Model file for the job. Use its own axes, mm. Give positions to 0.01 mm unless a question says otherwise; leave off trailing zeros. Loops run counter-clockwise (first coordinate to the right, second up) from the corner with the lowest first, then second, coordinate; pieces in that order, holes last. Notation, with made-up numbers: M 69,2.5 L 112,2.5 A28 ccw 112,33.5 Z; hole C 79,50 d2. An arc over 180 degrees is marked long. Use CSV: the item, a comma, the result in double quotes. Start each with the question number.
(1) Flat gauge pins, fed straight in: P1, Ø3, axis at x = 3, y = 407, coming from the -Z side; P2, Ø1.5, axis at x = 4.5, y = 323, coming from the -Z side; P3, Ø2, axis at x = 1, y = 427, coming from the -Z side. Where does each tip first touch, or does it go through?
(2) Slice it at D-D on z = 72.5. List the corners of the cut face in (x, y).
(3) Wall check: line 1 along Y through (x, z) = (2, 64); line 2 along Y through (x, z) = (0.5, 52); line 3 along Z through (x, y) = (1, 267.5). Give the ranges that are in metal, low to high. Write a range as from..to.
(4) Slice it at A-A on x = 5. List the corners of the cut face in (y, z).
(5) Slice it at B-B on z = 31.5. List the corners of the cut face in (x, y), and give its area (3 significant figures).
(6) Slice it at C-C on y = 269. List the corners of the cut face in (x, z).
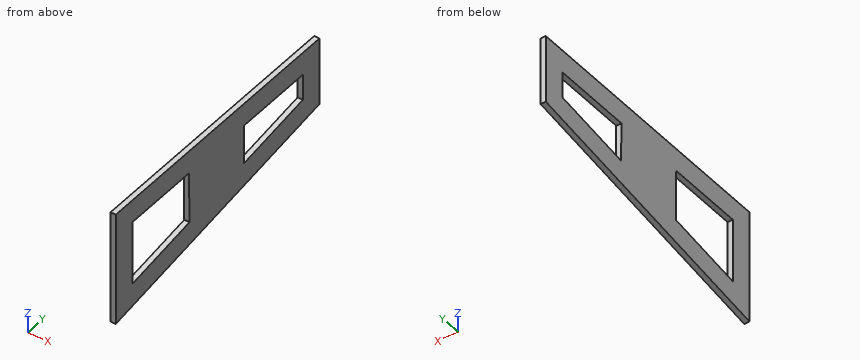
```python
from build123d import *

# Parameters (mm, degrees)
F1_DEPTH = 7


with BuildPart() as f1:
    # F0 (on Right) → F1 (new body)
    with BuildSketch(Plane.YZ):
        Polygon((599.109616, 110.551124), (232.423452, 105.89446), (232.423452, -44.10554), (599.109616, 20.551124), align=None)
        Polygon((262.423452, -8.352933), (262.423452, 76.27302), (364.232124, 77.565921), (365.093333, 9.750538), align=None, mode=Mode.SUBTRACT)
        Polygon((462.911965, 78.819088), (569.109616, 80.167725), (569.109616, 45.724113), (463.56858, 27.114381), align=None, mode=Mode.SUBTRACT)
    extrude(amount=F1_DEPTH)


solid = f1.part
```
Reply:
1,P1,"stops at z = -13.59"
1,P2,"stops at z = -28.27"
1,P3,"stops at z = -9.97"
2,outline,"M 0,232.42 L 7,232.42 L 7,262.42 L 0,262.42 Z; M 0,364.3 L 7,364.3 L 7,462.99 L 0,462.99 Z; M 0,569.11 L 7,569.11 L 7,599.11 L 0,599.11 Z"
3,line 1,"y = 232.42..262.42, 364.4..463.1, 569.11..599.11"
3,line 2,"y = 232.42..262.42, 364.56..463.25, 569.11..599.11"
3,line 3,"z = -37.92..-7.46, 76.34..106.34"
4,outline,"M 232.42,-44.11 L 599.11,20.55 L 599.11,110.55 L 232.42,105.89 Z; hole M 262.42,-8.35 L 365.09,9.75 L 364.23,77.57 L 262.42,76.27 Z; hole M 462.91,78.82 L 463.57,27.11 L 569.11,45.72 L 569.11,80.17 Z"
5,outline,"M 0,232.42 L 7,232.42 L 7,262.42 L 0,262.42 Z; M 0,364.82 L 7,364.82 L 7,463.51 L 0,463.51 Z; M 0,488.44 L 7,488.44 L 7,599.11 L 0,599.11 Z"
5,area,"1,680 mm^2"
6,outline,"M 0,-37.66 L 7,-37.66 L 7,-7.19 L 0,-7.19 Z; M 0,76.36 L 7,76.36 L 7,106.36 L 0,106.36 Z"
